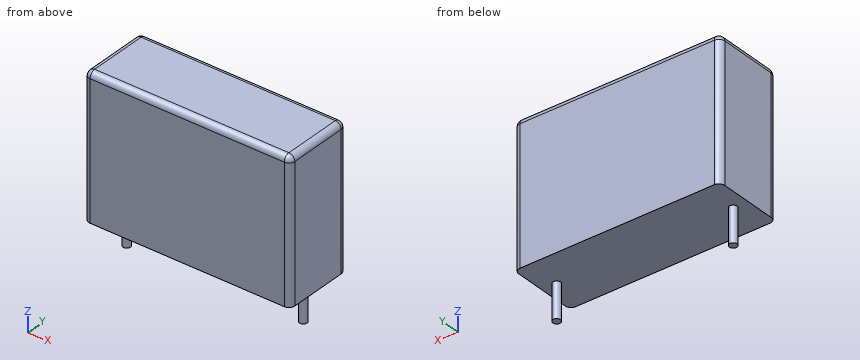
from build123d import *

# Parameters (mm, degrees)
CYLINDER001_R     = 0.33
CYLINDER001_DEPTH = 3
CYLINDER_R        = 0.33
CYLINDER_DEPTH    = 3
BOX_W             = 17.5
BOX_H             = 6
BOX_DEPTH         = 12
FILLET_R          = 0.5


with BuildPart() as pin2:
    # Cylinder001 → Cylinder001 (new body)
    with BuildSketch(Plane(origin=(7.5, 0, -3), x_dir=(1, 0, 0), z_dir=(0, 0, 1))):
        Circle(CYLINDER001_R)
    extrude(amount=CYLINDER001_DEPTH)


with BuildPart() as pin1:
    # Cylinder → Cylinder (new body)
    with BuildSketch(Plane(origin=(-7.5, 0, -3), x_dir=(1, 0, 0), z_dir=(0, 0, 1))):
        Circle(CYLINDER_R)
    extrude(amount=CYLINDER_DEPTH)


with BuildPart() as obj1:
    # Box → Box (new body)
    with BuildSketch(Plane(origin=(-8.75, -3, 0), x_dir=(1, 0, 0), z_dir=(0, 0, 1))):
        with Locations((8.75, 3)):
            Rectangle(BOX_W, BOX_H)
    extrude(amount=BOX_DEPTH)

    # Fillet
    fillet_edges = [obj1.edges().sort_by_distance(p)[0] for p in [
        (-8.75, -3, 6),
        (-8.75, 0, 12),
        (-8.75, 3, 6),
        (8.75, -3, 6),
        (8.75, 0, 12),
        (8.75, 3, 6),
        (0, -3, 12),
        (0, 3, 12),
    ]]
    fillet(fillet_edges, radius=FILLET_R)

    # Fusion: union Pin1
    add(pin1.part)

    # Fusion001: union Pin2
    add(pin2.part)


solid = obj1.part
Can you work these out from the model? Positions are in its coordinate system, mm. Round coordinates to 2 decimals unless told otherwise and drop trailing zeros. Order: outer loops, then holes, each group sorted by start corner. A loop starts at its lowest first (then second) coordinate and runs counter-clockwise, first axis right, second up. Notation, with made-up numbers: (63.25, -32) -> (109.25, -32) arc R19 ccw to (109.25, 5) -> close; hole circle Ø8 at (-26, 86). An arc over 180 degrees is marked (long way). Write each question's results on one line, items separated by ' | '. Start each with the question number.
Item 1: Please list where these lines run through material, in increasing order: L1, parallel to X at y = 0.05, z = -2; L2, parallel to Z at x = -4.75, y = 1.55; L3, parallel to X at y = -2.55, z = 8.
Item 2: If we section it at D-D, the plane y = -0.95: Write out the boundary of the cut face in (x, z).
Item 3: If we section it at A-A, the plane x = -7.5: Write out the boundary of the cut face in (y, z), then the cut area to 3 significant figures.
Item 4: If we section it at C-C, the plane x = -4.5: Write out the boundary of the cut face in (y, z).
Item 5: If we section it at B-B, the plane y = 0: Write out the boundary of the cut face in (x, z), then the cut area to 3 significant figures.
Results:
1) L1: x = -7.83 to -7.17, 7.17 to 7.83 | L2: z = 0 to 12 | L3: x = -8.75 to 8.75
2) outline: (-8.75, 0) -> (8.75, 0) -> (8.75, 11.5) arc R0.5 ccw to (8.25, 12) -> (-8.25, 12) arc R0.5 ccw to (-8.75, 11.5) -> close
3) outline: (-3, 0) -> (-0.33, 0) -> (-0.33, -3) -> (0.33, -3) -> (0.33, 0) -> (3, 0) -> (3, 11.5) arc R0.5 ccw to (2.5, 12) -> (-2.5, 12) arc R0.5 ccw to (-3, 11.5) -> close | area: 73.9 mm2
4) outline: (-3, 0) -> (3, 0) -> (3, 11.5) arc R0.5 ccw to (2.5, 12) -> (-2.5, 12) arc R0.5 ccw to (-3, 11.5) -> close
5) outline: (-8.75, 0) -> (-7.83, 0) -> (-7.83, -3) -> (-7.17, -3) -> (-7.17, 0) -> (7.17, 0) -> (7.17, -3) -> (7.83, -3) -> (7.83, 0) -> (8.75, 0) -> (8.75, 11.5) arc R0.5 ccw to (8.25, 12) -> (-8.25, 12) arc R0.5 ccw to (-8.75, 11.5) -> close | area: 214 mm2
